```python
from build123d import *
from OCP.BRepFilletAPI import BRepFilletAPI_MakeChamfer

# Parameters (mm, degrees)
BOSS_EXTRUDE1_DEPTH      = 10
SKETCH4_W                = 12.46
SKETCH4_H                = 17.25
BOSS_EXTRUDE3_DEPTH      = 6
BOSS_EXTRUDE6_DEPTH      = 7.3
BOSS_EXTRUDE6_DEPTH_BACK = 17.25
SKETCH8_R                = 12.546781182
SKETCH8_R_2              = 11.15
BOSS_EXTRUDE4_DEPTH      = 17.25
SKETCH6_R                = 2
CUT_EXTRUDE1_DEPTH       = 5
CHAMFER1_SIZE            = 0.5
CHAMFER1_SIZE_2          = 0.866025404
BOSS_EXTRUDE2_DEPTH      = 10
SKETCH10_W               = 12.46
SKETCH10_H               = 23.7
CUT_EXTRUDE3_DEPTH       = 17.25
CUT_EXTRUDE4_REACH       = 128.15
SKETCH11_W               = 5
SKETCH11_H               = 3
BOSS_EXTRUDE7_START      = -7.3
BOSS_EXTRUDE7_DEPTH      = 7.3


with BuildPart() as part:
    # Sketch1 → Boss-Extrude1 (new body)
    with BuildSketch(Plane.XY):
        Polygon((0, 0), (54.4906896, 75), (-54.4906896, 75), align=None)
    extrude(amount=BOSS_EXTRUDE1_DEPTH)

    # Sketch4 → Boss-Extrude3 (add)
    with BuildSketch(Plane.XY.offset(10)):
        with Locations((0, 63.875025481)):
            Rectangle(SKETCH4_W, SKETCH4_H)
    extrude(amount=BOSS_EXTRUDE3_DEPTH)



with BuildPart() as body_2:
    # Sketch8 → Boss-Extrude6 (new, two sides: drawn at the far end of the back side and taken through both)
    with BuildSketch(Plane(origin=(0, 55.250025481, 0), x_dir=(-1, 0, 0), z_dir=(0, -1, 0)).offset(-BOSS_EXTRUDE6_DEPTH_BACK)):
        with Locations(Location((0, -33.55, 0), (0, 0, 90))):
            Circle(SKETCH8_R)
        with Locations(Location((0, -33.55, 0), (0, 0, 90))):
            Circle(SKETCH8_R_2, mode=Mode.SUBTRACT)
    extrude(amount=BOSS_EXTRUDE6_DEPTH + BOSS_EXTRUDE6_DEPTH_BACK)


with BuildPart() as part_1:
    add(part.part)

    add(body_2.part)  # Boss-Extrude4 merges body 2
    # Sketch5 → Boss-Extrude4 (add)
    with BuildSketch(Plane(origin=(0, 72.500025481, 0), x_dir=(1, 0, 0), z_dir=(0, 1, 0))):
        with BuildLine():
            Line((12.546781182, -33.55), (12.546781182, -10))
            Line((12.546781182, -10), (6.23, -10))
            Line((6.23, -10), (6.23, -39.7))
            Line((6.23, -39.7), (-6.23, -39.7))
            Line((-6.23, -39.7), (-6.23, -10))
            Line((-6.23, -10), (-12.546781182, -10))
            Line((-12.546781182, -10), (-12.546781182, -33.55))
            ThreePointArc((-12.546781182, -33.55), (0, -46.096781182), (12.546781182, -33.55))
        make_face()
    extrude(amount=-BOSS_EXTRUDE4_DEPTH)

    # Sketch6 → Cut-Extrude1 (cut)
    with BuildSketch(Plane(origin=(0, 72.500025481, 0), x_dir=(1, 0, 0), z_dir=(0, 1, 0))):
        with Locations(Location((0, -13.5, 0), (0, 0, 270))):
            Circle(SKETCH6_R)
        with Locations(Location((0, -42.2, 0), (0, 0, 270))):
            Circle(SKETCH6_R)
    extrude(amount=-CUT_EXTRUDE1_DEPTH, mode=Mode.SUBTRACT)

    # Chamfer1
    chamfer1_edges_1 = [part_1.edges().sort_by_distance(p)[0] for p in [
        (0, 72.500025481, 11.5),
    ]]
    chamfer1_side_1 = [part_1.faces().sort_by_distance(p)[0] for p in [
        (0, 72.500025481, 11.49),
    ]]
    chamfer1_edges_2 = [part_1.edges().sort_by_distance(p)[0] for p in [
        (0, 72.500025481, 40.2),
    ]]
    chamfer1_side_2 = [part_1.faces().sort_by_distance(p)[0] for p in [
        (0, 72.500025481, 40.19),
    ]]
    chamfer1 = BRepFilletAPI_MakeChamfer(part_1.part.solid().wrapped)
    for e in chamfer1_edges_1:
        chamfer1.Add(CHAMFER1_SIZE - 0.0001, CHAMFER1_SIZE_2 - 0.0001, e.wrapped, chamfer1_side_1[0].wrapped)
    for e in chamfer1_edges_2:
        chamfer1.Add(CHAMFER1_SIZE - 0.0001, CHAMFER1_SIZE_2 - 0.0001, e.wrapped, chamfer1_side_2[0].wrapped)
    add(Compound.cast(chamfer1.Shape()), mode=Mode.REPLACE)  # a hair under: the kernel refuses the full size

    # Sketch2 → Boss-Extrude2 (add)
    with BuildSketch(Plane.XY):
        Polygon((-54.4906896, 75), (-69.021540161, 95), (69.021540161, 95), (54.4906896, 75), align=None)
    extrude(amount=BOSS_EXTRUDE2_DEPTH)

    # Sketch10 → Cut-Extrude3 (cut)
    with BuildSketch(Plane(origin=(0, 72.500025481, 0), x_dir=(1, 0, 0), z_dir=(0, 1, 0))):
        with Locations((0, -27.85)):
            Rectangle(SKETCH10_W, SKETCH10_H)
    extrude(amount=-CUT_EXTRUDE3_DEPTH, mode=Mode.SUBTRACT)

    # Sketch11 → Cut-Extrude4 (cut, up to next)
    with BuildSketch(Plane.XY.offset(46.096781182), mode=Mode.PRIVATE) as cut_extrude4_sk1:
        with Locations((0, 56.750025481)):
            Rectangle(SKETCH11_W, SKETCH11_H)
    cut_extrude4_tool1 = extrude(cut_extrude4_sk1.sketch, amount=-CUT_EXTRUDE4_REACH, mode=Mode.PRIVATE) & part_1.part
    add(cut_extrude4_tool1.solids().sort_by_distance((0, 56.750025, 46.096781))[0], mode=Mode.SUBTRACT)

    # Sketch13 → Boss-Extrude7 (add)
    with BuildSketch(Plane.XZ.offset(-47.950025481).offset(BOSS_EXTRUDE7_START)):
        with BuildLine():
            Line((-12.546781182, 33.55), (-12.546781182, 10))
            Line((-12.546781182, 10), (12.546781182, 10))
            Line((12.546781182, 10), (12.546781182, 33.55))
            ThreePointArc((12.546781182, 33.55), (0, 21.003218818), (-12.546781182, 33.55))
        make_face()
    extrude(amount=BOSS_EXTRUDE7_DEPTH)


solid = part_1.part
```
Source: CAD feature listing. Evaluate the final solid. Frame: model axes, mm. A direction names the side the tool comes from. Give positions to 0.01 mm unless a question says otherwise; leave off trailing zeros. Write each loop counter-clockwise with the first axis right and the second up, starting at its lowest first coordinate (ties: lowest second). Pieces come first, ordered by that corner, then holes.
1. Section query C-C (y = 21). Return the cut outline in (x, z).
2. Section query D-D (z = 6.5). Return the cut outline in (x, y), then the cut area to 3 significant figures.
3. Section query B-B (x = -59). Return the cut outline in (y, z).
4. Material intervals for line 1 along X through (y, z) = (49, 33); line 2 along X through (y, z) = (71, 19); line 3 along Z through (x, y) = (0, 50), sorted ascending.
5. Pull-direction query (X, two-part tool) for faces 4 (the face through (-9, 72.5, 28)), 5 (the face through (-1.2, 69.6, 11.9)), 6 (the face through (-12.547, 60, 22)); classes: +X half, -X half, draft (parallel to the pull), parting line (faces both ways), or undercut.
6. Access query for faces 1 (the face through (0, 58.25, 43)), 2 (the face through (0, 67.5, 42)), 3 (the face through (3.3, 51.7, 22.9)). Directions: +Z, -Z, +X, -X, +Y, -Y. A direction counts if a zero-diameter tool reaches every point of the face in a straight line with its end or side. Return the directions, or none.
7. First-contact query: pin 1 (3.5 mm diameter, centred on x = 0.5, y = 64, fed in from +Z); pin 2 (6 mm diameter, centred on y = 51.5, z = 22.5, fed in from +X); pin 3 (7.5 mm diameter, centred on y = 67.5, z = 35.5, fed in from -X); pin 4 (2.5 mm diameter, centred on x = 0, z = 23, fed in from +Y). Flat tips, straight axial feed; report the tip coordinate or a pass-through.
8. Section query A-A (z = 13.5). Return the cut outline in (x, y), then the cut area to 3 significant figures.
Output values:
1. outline: (-15.26, 0) - (15.26, 0) - (15.26, 10) - (-15.26, 10) - close
2. outline: (-69.02, 95) - (0, 0) - (69.02, 95) - close
2. area: 6,560 mm2
3. outline: (81.21, 0) - (95, 0) - (95, 10) - (81.21, 10) - close
4. line 1: x = -12.55 to -11.14, 11.14 to 12.55
4. line 2: x = -12.55 to -6.23, 6.23 to 12.55
4. line 3: z = 0 to 22.4, 44.7 to 46.1
5. face 4: draft
5. face 5: undercut
5. face 6: -X half
6. face 1: +Z
6. face 2: +Y
6. face 3: -Y
7. pin 1: stops at z = 46.1
7. pin 2: stops at x = 12.55
7. pin 3: stops at x = -12.55
7. pin 4: stops at y = 55.25
8. outline: (-12.55, 47.95) - (12.55, 47.95) - (12.55, 72.5) - (2.5, 72.5) - (2, 71.63) - (2, 67.5) - (-2, 67.5) - (-2, 71.63) - (-2.5, 72.5) - (-12.55, 72.5) - close
8. area: 596 mm2
